Here's how the part is built. I have some questions about the finished solid (model axes, mm). A direction names the side the tool comes from. Give positions to 0.01 mm unless a question says otherwise; leave off trailing zeros. Loops run counter-clockwise (first coordinate to the right, second up) from the corner with the lowest first, then second, coordinate; pieces in that order, holes last. Notation, with made-up numbers: (6.25, -37) - (56.25, -37) arc R16 cw to (56.25, -24) - close; hole circle Ø4 at (-35.75, 57.25). An arc over 180 degrees is marked (long way). Use one line per item in the form item = value.
from build123d import *

# Parameters (mm, degrees)
BOSS_EXTRUDE1_DEPTH     = 10
CUT_EXTRUDE1_DEPTH      = 72.414284285
CUT_EXTRUDE1_DEPTH_BACK = 72.414284285
SKETCH2_R               = 1.5
SKETCH9_W               = 10
SKETCH9_H               = 50
BOSS_EXTRUDE9_DEPTH     = 5
SKETCH10_W              = 10
SKETCH10_H              = 50
BOSS_EXTRUDE10_DEPTH    = 5
BOSS_EXTRUDE11_DEPTH    = 2
SKETCH12_W              = 10
SKETCH12_H              = 10
BOSS_EXTRUDE12_DEPTH    = 5
CUT_EXTRUDE2_START      = 7
SKETCH13_R              = 1.5
CUT_EXTRUDE2_DEPTH      = 7
BOSS_EXTRUDE13_DEPTH    = 2
SKETCH15_W              = 9.981523119
SKETCH15_H              = 10
BOSS_EXTRUDE14_DEPTH    = 30
SKETCH16_R              = 1.5
CUT_EXTRUDE3_DEPTH      = 32
SKETCH17_W              = 110
SKETCH17_H              = 63.73964009
BOSS_EXTRUDE15_DEPTH    = 10
CUT_EXTRUDE4_REACH      = 83.695
SKETCH18_W              = 100.013857661
SKETCH18_H              = 2
SKETCH19_W              = 90.018476881
SKETCH19_H              = 50
CUT_EXTRUDE5_DEPTH      = 10
CUT_EXTRUDE6_DEPTH      = 80.837334625
SKETCH21_W              = 90.018476881
SKETCH21_H              = 30.73964009
CUT_EXTRUDE7_DEPTH      = 80.837334625
FILLET1_R               = 5
FILLET2_R               = 15
FILLET3_R               = 5


with BuildPart() as part:
    # Sketch1 → Boss-Extrude1 (new body)
    with BuildSketch(Plane.XY):
        with BuildLine():
            Line((45.018476881, -25), (50, -25))
            Line((50, -25), (50, 25))
            Line((50, 25), (45, 25))
            ThreePointArc((45, 25), (0, 8), (-45, 25))
            Line((-45, 25), (-50, 25))
            Line((-50, 25), (-50, -25))
            Line((-50, -25), (-45.018476881, -25))
            ThreePointArc((-45.018476881, -25), (0, -8), (45.018476881, -25))
        make_face()
    extrude(amount=BOSS_EXTRUDE1_DEPTH)

    # Sketch2 → Cut-Extrude1 (cut, two sides: drawn at the far end of the back side and taken through both)
    with BuildSketch(Plane(origin=(0, 25, 0), x_dir=(1, 0, 0), z_dir=(0, 1, 0)).offset(-CUT_EXTRUDE1_DEPTH_BACK)):
        with Locations(Location((-48, -5, 0), (0, 0, 180))):
            Circle(SKETCH2_R)
        with Locations(Location((48, -5, 0), (0, 0, 180))):
            Circle(SKETCH2_R)
    extrude(amount=CUT_EXTRUDE1_DEPTH + CUT_EXTRUDE1_DEPTH_BACK, mode=Mode.SUBTRACT)

    # Sketch9 → Boss-Extrude9 (add)
    with BuildSketch(Plane(origin=(50, 0, 0), x_dir=(0, 0, -1), z_dir=(1, 0, 0))):
        with Locations((-5, 0)):
            Rectangle(SKETCH9_W, SKETCH9_H)
    extrude(amount=BOSS_EXTRUDE9_DEPTH)

    # Sketch10 → Boss-Extrude10 (add)
    with BuildSketch(Plane.ZY.offset(50)):
        with Locations((5, 0)):
            Rectangle(SKETCH10_W, SKETCH10_H)
    extrude(amount=BOSS_EXTRUDE10_DEPTH)

    # Sketch11 → Boss-Extrude11 (add)
    with BuildSketch(Plane(origin=(0, 25, 0), x_dir=(1, 0, 0), z_dir=(0, 1, 0))):
        Polygon((50, 0), (50, -7), (45, -7), (45, -10), (55, -10), (55, 0), align=None)
        Polygon((-50, 0), (-50, -7), (-45, -7), (-45, -10), (-55, -10), (-55, 0), align=None)
    extrude(amount=BOSS_EXTRUDE11_DEPTH)

    # Sketch12 → Boss-Extrude12 (add)
    with BuildSketch(Plane(origin=(0, 27, 0), x_dir=(1, 0, 0), z_dir=(0, 1, 0))):
        with Locations((50, -5)):
            Rectangle(SKETCH12_W, SKETCH12_H)
        with Locations((-50, -5)):
            Rectangle(SKETCH12_W, SKETCH12_H)
    extrude(amount=BOSS_EXTRUDE12_DEPTH)

    # Sketch13 → Cut-Extrude2 (cut)
    with BuildSketch(Plane(origin=(0, 25, 0), x_dir=(1, 0, 0), z_dir=(0, 1, 0)).offset(CUT_EXTRUDE2_START)):
        with Locations(Location((48, -5, 0), (0, 0, 180))):
            Circle(SKETCH13_R)
        with Locations(Location((-48, -5, 0), (0, 0, 180))):
            Circle(SKETCH13_R)
    extrude(amount=-CUT_EXTRUDE2_DEPTH, mode=Mode.SUBTRACT)

    # Sketch14 → Boss-Extrude13 (add)
    with BuildSketch(Plane.XZ.offset(25)):
        Polygon((50.009238441, 0), (50.009238441, 7), (45.018476881, 7), (45.018476881, 10), (55, 10), (55, 0), align=None)
        Polygon((-50.009238441, 0), (-50.009238441, 7), (-45.018476881, 7), (-45.018476881, 10), (-55, 10), (-55, 0), align=None)
    extrude(amount=BOSS_EXTRUDE13_DEPTH)

    # Sketch15 → Boss-Extrude14 (add)
    with BuildSketch(Plane.XZ.offset(27)):
        with Locations((-50.00923844, 5)):
            Rectangle(SKETCH15_W, SKETCH15_H)
        with Locations((50.00923844, 5)):
            Rectangle(SKETCH15_W, SKETCH15_H)
    extrude(amount=BOSS_EXTRUDE14_DEPTH)

    # Sketch16 → Cut-Extrude3 (cut)
    with BuildSketch(Plane.XZ.offset(25)):
        with Locations(Location((48, 5, 0), (0, 0, 180))):
            Circle(SKETCH16_R)
        with Locations(Location((-48, 5, 0), (0, 0, 180))):
            Circle(SKETCH16_R)
    extrude(amount=CUT_EXTRUDE3_DEPTH, mode=Mode.SUBTRACT)

    # Sketch17 → Boss-Extrude15 (add)
    with BuildSketch(Plane.XY.offset(10)):
        with Locations((0, 0.130179955)):
            Rectangle(SKETCH17_W, SKETCH17_H)
    extrude(amount=BOSS_EXTRUDE15_DEPTH)

    # Cut-Extrude4: up to this face of the body (flat: up to its plane)
    cut_extrude4_end = Plane(part.part.faces().sort_by_distance((47.5, 26, 7))[0])
    # Sketch18 → Cut-Extrude4 (cut, up to the picked face)
    with BuildSketch(Plane(origin=(0, 0, 0), x_dir=(-1, 0, 0), z_dir=(0, 0, -1)), mode=Mode.PRIVATE) as cut_extrude4_sk1:
        with Locations((-0.00230961, 0)):
            Rectangle(SKETCH18_W, SKETCH18_H)
    cut_extrude4_tool1 = split(extrude(cut_extrude4_sk1.sketch, amount=-CUT_EXTRUDE4_REACH, mode=Mode.PRIVATE), bisect_by=cut_extrude4_end, keep=Keep.BOTH, mode=Mode.PRIVATE)
    add(cut_extrude4_tool1.solids().sort_by(Axis((0.00231, 0, 0), (0, 0, 1)))[0], mode=Mode.SUBTRACT)

    # Sketch19 → Cut-Extrude5 (cut)
    with BuildSketch(Plane(origin=(0, 0, 0), x_dir=(-1, 0, 0), z_dir=(0, 0, -1))):
        with Locations((-0.009238441, 0)):
            Rectangle(SKETCH19_W, SKETCH19_H)
    extrude(amount=-CUT_EXTRUDE5_DEPTH, mode=Mode.SUBTRACT)

    # Sketch20 → Cut-Extrude6 (cut, through all)
    with BuildSketch(Plane(origin=(0, 0, 10), x_dir=(-1, 0, 0), z_dir=(0, 0, -1))):
        with BuildLine():
            Line((-45, 32), (45, 32))
            ThreePointArc((45, 32), (0, 13.452072887), (-45, 32))
        make_face()
    extrude(amount=-CUT_EXTRUDE6_DEPTH, mode=Mode.SUBTRACT)

    # Sketch21 → Cut-Extrude7 (cut, through all)
    with BuildSketch(Plane(origin=(0, 0, 10), x_dir=(-1, 0, 0), z_dir=(0, 0, -1))):
        with Locations((-0.009238441, -16.369820045)):
            Rectangle(SKETCH21_W, SKETCH21_H)
    extrude(amount=-CUT_EXTRUDE7_DEPTH, mode=Mode.SUBTRACT)

    # Fillet1
    fillet1_edges = [part.edges().sort_by_distance(p)[0] for p in [
        (50.009238441, -31.73964009, 20),
        (50.009238441, -31.73964009, 10),
        (-50, -31.73964009, 20),
        (-50.009238441, -31.73964009, 10),
    ]]
    fillet(fillet1_edges, radius=FILLET1_R - 0.0001)  # a hair under: the kernel refuses the full size

    # Fillet2
    fillet2_edges = [part.edges().sort_by_distance(p)[0] for p in [
        (45.018476881, -1, 15),
        (-45, -1, 15),
    ]]
    fillet(fillet2_edges, radius=FILLET2_R)

    # Fillet3
    fillet3_edges = [part.edges().sort_by_distance(p)[0] for p in [
        (-55, 2.630129955, 20),
        (55, 2.630129955, 20),
        (55, -46.869770045, 10),
        (55, -30.275203285, 18.535563195),
        (-55, -30.275203285, 18.535563195),
        (55, -33.204076895, 11.464436805),
        (-55, -33.204076895, 11.464436805),
        (-55, -46.869770045, 10),
    ]]
    fillet(fillet3_edges, radius=FILLET3_R - 0.0001)  # a hair under: the kernel refuses the full size


solid = part.part
(1) Thinking about a two-plate mould opening in Y: for faces 4 (the flat face through (50, -57, 5)), 5 (the cylindrical face through (49.5, 12.83, 5.07)), 6 (the flat face through (47, 27, 3)), which applies, pulls with the +Y half, pulls with the -Y half, needs draft (parallel to the pull), parting line crosses it, or undercut?
Geometry says:
face_4 = pulls with the -Y half
face_5 = needs draft
face_6 = undercut
(2) For faces 1 (the flat face through (45, 29, 5)), 2 (the flat face through (47, -27, 3)), 3 (the cylindrical face through (53, -47, 9)), which set-ups out of +Z, -Z, +X, -X, +Y, -Y let a thin tool reach every point of the face, with its end or its side?
Geometry says:
face_1 = -Z, +Y, -Y
face_2 = -Z
face_3 = +Z, +X, -Y
(3) If I drill on probe 1 along X at (y, z) = (-40.5, 5); probe 2 along Z at (x, y) = (48, -13.5); probe 3 along Z at (x, y) = (48, -49), over which ranges is the centre line in solid material (lowest first)?
Geometry says:
probe_1 = -55 to -49.5, -46.5 to -45.02, 45.02 to 46.5, 49.5 to 55
probe_2 = 0 to 3.5, 6.5 to 20
probe_3 = 0 to 3.5, 6.5 to 10
(4) If we section it at A-A (y = -45): List the corners of the cut face in (x, z) for me.
Geometry says:
outline = (-55, 0) - (-45.02, 0) - (-45.02, 10) - (-50, 10) arc R5 ccw to (-55, 5) - close; (45.02, 0) - (55, 0) - (55, 5) arc R5 ccw to (50, 10) - (45.02, 10) - close; hole circle Ø3 at (-48, 5); hole circle Ø3 at (48, 5)
(5) If we section it at D-D (z = 16.75): List the corners of the cut face in (x, y) for me, plus the area to 3 significant figures.
Geometry says:
outline = (-54.68, -26.74) arc R4.68 ccw to (-50, -31.42) - (-45, -31.42) - (-45, -16) arc R15 cw to (-30, -1) - (30.02, -1) arc R15 cw to (45.02, -16) - (45.02, -31.42) - (50, -31.42) arc R4.68 ccw to (54.68, -26.74) - (54.68, 32) - (45, 32) arc R63.86 cw to (-45, 32) - (-54.68, 32) - close
area = 3,140 mm²
(6) If we section it at C-C (x = 48): Give the number of separate pieces and of enclosed holes in the cut face, plus the area to 3 significant figures.
Geometry says:
separate_pieces = 5
enclosed_holes = 0
area = 1,240 mm²
(7) For P1, Ø6, axis at x = -22.5, z = 12, coming from the +Y side; P2, Ø1.6, axis at x = 47.5, y = 26, coming from the -Z side; P3, Ø4, axis at x = -32, z = 10.5, coming from the +Y side, each with a flat end and sliding along its axis, tell me the tip position at first contact or that it passes through.
Geometry says:
P1 = 18.76
P2 = 7
P3 = 23.26
